Input: part model. Units: mm. Frame: model coordinates. Round coordinates to 2 decimals unless told otherwise and drop trailing zeros. Loops run counter-clockwise (first coordinate to the right, second up) from the corner with the lowest first, then second, coordinate; pieces in that order, holes last. Notation, with made-up numbers: M -20.75,18 L 30.25,18 A22 cw 30.25,24 Z; hole C 82,34.25 d8. An arc over 180 degrees is marked long. Put each result on its own line as item: value. Start each with the question number.
1) Section D-D on x = 60.5. Output: boundary loops of the cut face in (y, z).
2) Section A-A on z = 0. Output: boundary loops of the cut face in (x, y).
3) Line query: probe 1 along Z at (x, y) = (-13, 1.2); probe 2 along X at (y, z) = (1.55, -9); probe 3 along X at (y, z) = (0.7, -16.5). Output: solid intervals per line, ascending.
4) Section B-B on x = 0. Output: boundary loops of the cut face in (y, z).
5) Section C-C on y = 0.75. Output: boundary loops of the cut face in (x, z), plus the area to 3 significant figures.
6) Pin query (flat end, axial travel): pin 1 (1.5 mm diameter, centred on x = 60.5, y = 2, fed in from -Z). Return the tip coordinate at first contact, or that it passes through.
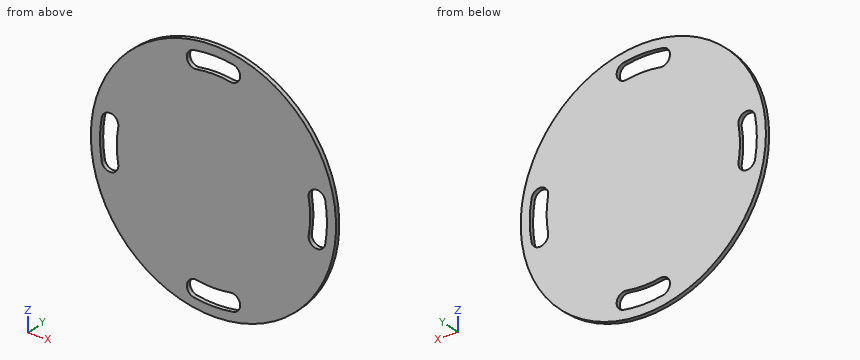
Autodesk Inventor part; units mm, degrees
ref_plane "YZ Plane" through (0, 0, 0) normal (1, 0, 0) x (0, 1, 0)
ref_plane "XZ Plane" through (0, 0, 0) normal (0, 1, 0) x (-1, 0, 0)
ref_plane "XY Plane" through (0, 0, 0) normal (0, 0, 1) x (1, 0, 0)
sketch "Sketch1" plane through (0, 0, 0) normal (0, 1, 0) x (-1, 0, 0)
  circle A0 centre (0, 0) radius 87.5
  dimension "d0" = 175
extrude "Plate1" add sketch "Sketch1" along normal blind 3
sketch "Sketch2" plane through (0, 3, 0) normal (0, 1, 0) x (1, 0, 0)
  circle A0 centre (0, 0) radius 87.5
  arc A1 (73.8606, -13.0236) -> (73.8606, 13.0236) centre (0, 0) ccw construction
  arc A2 (79.7694, -14.0655) -> (79.7694, 14.0655) centre (0, 0) ccw
  arc A3 (67.9517, -11.9817) -> (67.9517, 11.9817) centre (0, 0) ccw
  arc A4 (67.9517, -11.9817) -> (79.7694, -14.0655) centre (73.8606, -13.0236) ccw
  arc A5 (79.7694, 14.0655) -> (67.9517, 11.9817) centre (73.8606, 13.0236) ccw
  point P0 (75, 0)
  dimension "d19" = 12
  dimension "d20" = 20
  dimension "d21" = 75
extrude "Extrusion1" cut sketch "Sketch2" against normal through all contours A4 A3 A5 A2
pattern_circular "Circular Pattern1" count 4 over 360 about axis through (0, -10, 0) along (0, 1, 0) of "Extrusion1"
equation "\"BendReliefWidth\" = Thickness"
equation "\"BendReliefDepth\" = 0.5 * Thickness"
equation "\"CornerReliefSize\" = 4 * Thickness"
equation "\"MinimumRemnant\" = 2 * Thickness"
equation "\"TransitionRadius\" = BendRadius"
equation "\"JacobiRadiusSize\" = BendRadius"
equation "\"GapSize\" = Thickness"
properties part number "MSC 906 flange frame" material "Stainless Steel"
Geometry results:
1. outline: M 0,-63.21 L 3,-63.21 L 3,63.21 L 0,63.21 Z
2. outline: M -87.5,0 L -81,0 L -81,3 L -87.5,3 Z; M -69,0 L 69,0 L 69,3 L -69,3 Z; M 81,0 L 87.5,0 L 87.5,3 L 81,3 Z
3. probe 1: z = -86.53 to -79.95, -67.86 to 67.86, 79.95 to 86.53
3. probe 2: x = -87.04 to -80.5, -68.41 to 68.41, 80.5 to 87.04
3. probe 3: x = -85.93 to -78.75, -68.97 to 68.97, 78.75 to 85.93
4. outline: M 0,-87.5 L 3,-87.5 L 3,-81 L 0,-81 Z; M 0,-69 L 3,-69 L 3,69 L 0,69 Z; M 0,81 L 3,81 L 3,87.5 L 0,87.5 Z
5. outline: C 0,0 d175; hole M -79.77,-14.07 A6 ccw -67.95,-11.98 A69 cw -67.95,11.98 A6 ccw -79.77,14.07 A81 ccw Z; hole M -14.07,-79.77 A81 ccw 14.07,-79.77 A6 ccw 11.98,-67.95 A69 cw -11.98,-67.95 A6 ccw Z; hole M -14.07,79.77 A6 ccw -11.98,67.95 A69 cw 11.98,67.95 A6 ccw 14.07,79.77 A81 ccw Z; hole M 67.95,-11.98 A6 ccw 79.77,-14.07 A81 ccw 79.77,14.07 A6 ccw 67.95,11.98 A69 cw Z
5. area: 22,300 mm²
6. pin 1: stops at z = -63.92
